Work out the finished part from the listing and answer in its coordinate system (mm). A direction names the side the tool comes from. Give positions to 0.01 mm unless a question says otherwise; leave off trailing zeros. Loops run counter-clockwise (first coordinate to the right, second up) from the corner with the lowest first, then second, coordinate; pieces in that order, holes last. Notation, with made-up numbers: M 34.25,32.25 L 85.25,32.25 A10 cw 85.25,37.25 Z; hole C 15.5,86 d11. An arc over 180 degrees is marked long. Answer in a Markdown table with one row per item. Add a question column.
from build123d import *

# Parameters (mm, degrees)
BOSS_EXTRUDE1_DEPTH = 2
SKETCH2_R           = 2
BOSS_EXTRUDE2_DEPTH = 2
BOSS_EXTRUDE3_DEPTH = 3
SKETCH4_R           = 1.5
BOSS_EXTRUDE4_DEPTH = 8


with BuildPart() as part:
    # Sketch1 → Boss-Extrude1 (new body)
    with BuildSketch(Plane(origin=(0, 0, 0), x_dir=(1, 0, 0), z_dir=(0, 1, 0))):
        Polygon((-12, -2), (-12, 2), (-8, 8), (0, 8), (0, -8), (-8, -8), align=None)
    extrude(amount=BOSS_EXTRUDE1_DEPTH)

    # Sketch2 → Boss-Extrude2 (add)
    with BuildSketch(Plane(origin=(0, 2, 0), x_dir=(1, 0, 0), z_dir=(0, 1, 0))):
        with Locations((-4, 4)):
            Circle(SKETCH2_R)
        with Locations((-4, -4)):
            Circle(SKETCH2_R)
    extrude(amount=BOSS_EXTRUDE2_DEPTH)

    # Sketch3 → Boss-Extrude3 (add)
    with BuildSketch(Plane(origin=(0, 2, 0), x_dir=(1, 0, 0), z_dir=(0, 1, 0))):
        Polygon((-12, -2), (-8, -8), (-8, -6.197224362), (-11, -1.697224362), (-11, 1.697224362), (-8, 6.197224362), (-8, 8), (-12, 2), align=None)
    extrude(amount=BOSS_EXTRUDE3_DEPTH)

    # Sketch4 → Boss-Extrude4 (add)
    with BuildSketch(Plane.ZY.offset(12)):
        with Locations((0, 2.5)):
            Circle(SKETCH4_R)
    extrude(amount=BOSS_EXTRUDE4_DEPTH)

    # Mirror2: part across plane


with BuildPart() as part_1:
    add(part.part)
    add(part.part.mirror(Plane(origin=(0, 0, 0), x_dir=(0, 0, 1), z_dir=(1, 0, 0))))


solid = part_1.part
(1) The mould has two halves that part along Z. Classify faces 1 (the face through (11, 3, 0)), 2 (the face through (-8, 3, 7)), 3 (the face through (10, 2, -5)), 4 (the face through (-5.6, 3, 5.2)): pulls with the +Z half, pulls with the -Z half, needs draft (parallel to the pull), parting line crosses it, or undercut.
(2) Each of these flat-tipped pins is pushed along its axis until it touches: P1, Ø3, axis at x = 5, z = -5, coming from the +Y side; P2, Ø0.9, axis at y = 3, z = -7, coming from the +X side; P3, Ø2, axis at y = 4, z = -7, coming from the -X side. Where does it stop, or does it pass through?
(3) Section B-B, the plane x = 4 is taken. Determine the outline of the cut face in (y, z), and give its area (3 significant figures).
(4) Section C-C, the plane z = 0 is taken. Determine the outline of the cut face in (x, y).
(5) Consider line 1 along X through (y, z) = (2.15, 3); line 2 along X through (y, z) = (3.7, -5.5); line 3 along X through (y, z) = (3.45, -0.75). Determine where each line is inside the solid, lowest interval first. Write a range as from..to.
(6) Section D-D, the plane x = -5.5 is taken. Determine the outline of the cut face in (y, z), and give its area (3 significant figures).
(7) Which of the six approach directions +Z, -Z, +X, -X, +Y, -Y give full straight-line access (tool end or side, diameter ignored) to faces 5 (the face through (12, 0.8, 0)), 6 (the face through (5.6, 3, -2.8)), 7 (the face through (-8, 3, -7))?
(8) Section A-A, the plane y = 2.5 is taken. Determine the outline of the cut face in (x, z), and give its area (3 significant figures).
Numbers:
| question | item | result |
|---|---|---|
| 1 | face 1 | undercut |
| 1 | face 2 | needs draft |
| 1 | face 3 | pulls with the -Z half |
| 1 | face 4 | undercut |
| 2 | P1 | stops at y = 4 |
| 2 | P2 | stops at x = 8.97 |
| 2 | P3 | stops at x = -9.33 |
| 3 | outline | M 0,-8 L 2,-8 L 2,-6 L 4,-6 L 4,-2 L 2,-2 L 2,2 L 4,2 L 4,6 L 2,6 L 2,8 L 0,8 Z |
| 3 | area | 48.0 mm² |
| 4 | outline | M -20,1 L -12,1 L -12,0 L 12,0 L 12,1 L 20,1 L 20,4 L 12,4 L 12,5 L 11,5 L 11,2 L -11,2 L -11,5 L -12,5 L -12,4 L -20,4 Z |
| 5 | line 1 | x = -11.33..-10.13, -5.73..-2.27, 2.27..5.73, 10.13..11.33 |
| 5 | line 2 | x = -9.67..-8.46, -5.32..-2.68, 2.68..5.32, 8.46..9.67 |
| 5 | line 3 | x = -20..-11, 11..20 |
| 6 | outline | M 0,-8 L 2,-8 L 2,-5.32 L 4,-5.32 L 4,-2.68 L 2,-2.68 L 2,2.68 L 4,2.68 L 4,5.32 L 2,5.32 L 2,8 L 0,8 Z |
| 6 | area | 42.6 mm² |
| 7 | face 5 | +X |
| 7 | face 6 | +Y |
| 7 | face 7 | +Z, -Z, +Y |
| 8 | outline | M -20,-1.5 L -12,-1.5 L -12,-2 L -8,-8 L -8,-6.2 L -11,-1.7 L -11,1.7 L -8,6.2 L -8,8 L -12,2 L -12,1.5 L -20,1.5 Z; C -4,-4 d4; C -4,4 d4; C 4,-4 d4; C 4,4 d4; M 8,-8 L 12,-2 L 12,-1.5 L 20,-1.5 L 20,1.5 L 12,1.5 L 12,2 L 8,8 L 8,6.2 L 11,1.7 L 11,-1.7 L 8,-6.2 Z |
| 8 | area | 131 mm² |
